Design review of the part shown in the three views and the two pictorial views. Dimensions are in mm from the part's minimum x, y and z. A direction names the side the tool comes from. Coordinates: 2 decimals unless noted, no trailing zeros. Loops run counter-clockwise (first coordinate to the right, second up) from the corner with the lowest first, then second, coordinate; pieces in that order, holes last. Notation, with made-up numbers: (28, 87.25) -> (53, 87.25) arc R21 cw to (53, 124.25) -> close; hole circle Ø6 at (47, 45.5). An arc over 180 degrees is marked (long way). One line per item, written item: value.
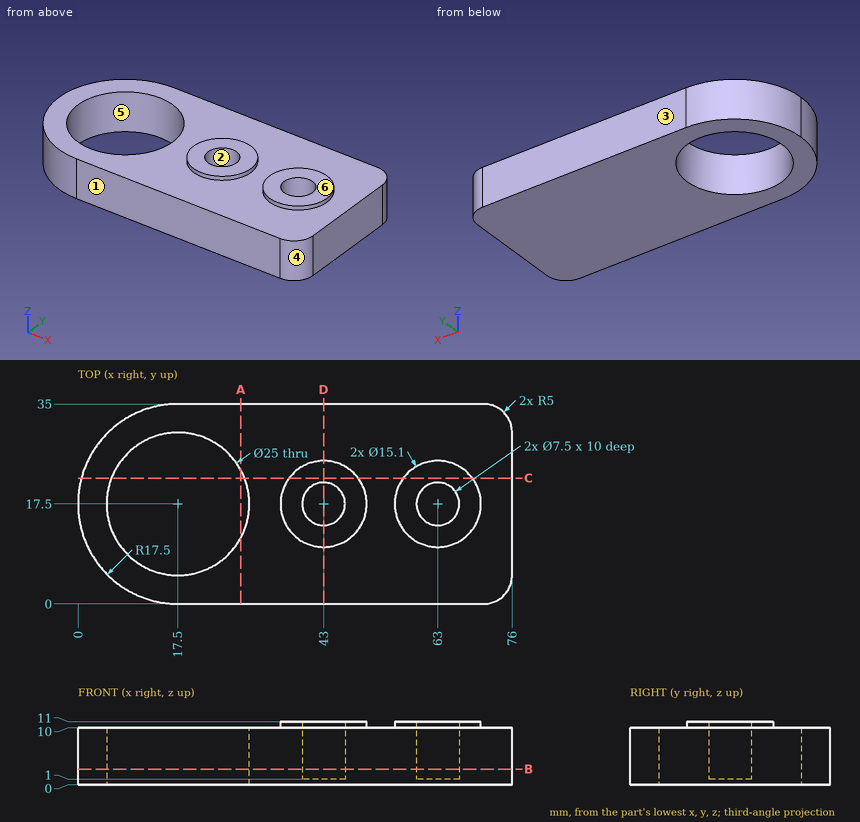
1. Insertion check: pin 1 Ø10.5 at (x, y) = (54, 11) entering from +Z; pin 2 Ø4 at (x, y) = (42.5, 18) entering from +Z; pin 3 Ø5 at (y, z) = (10.5, 3) entering from -X; pin 4 Ø6 at (y, z) = (11, 2) entering from -X. Each pin has a flat end and moves straight along its axis. Give the tip position at first contact, or say it passes through.
Return value:
pin 1: stops at z = 11
pin 2: stops at z = 1
pin 3: stops at x = 0.59
pin 4: stops at x = 0.35
2. Take a section at D-D, the plane x = 43. Give the boundary of the cut face in (y, z), and give its area (3 significant figures).
Return value:
outline: (0, 0) -> (35, 0) -> (35, 10) -> (25.05, 10) -> (25.05, 11) -> (21.25, 11) -> (21.25, 1) -> (13.75, 1) -> (13.75, 11) -> (9.95, 11) -> (9.95, 10) -> (0, 10) -> close
area: 290 mm2
3. The part is to be moulded in two halves that separate along Y. For the marked faces 3, 4, 5 and 6, say which applies: pulls with the +Y half, pulls with the -Y half, needs draft (parallel to the pull), parting line crosses it, or undercut.
Return value:
face 3: pulls with the +Y half
face 4: pulls with the -Y half
face 5: undercut
face 6: needs draft
4. Take a section at B-B, the plane z = 2.75. Give the boundary of the cut face in (x, y), and give its area (3 significant figures).
Return value:
outline: (17.5, 0) -> (71, 0) arc R5 ccw to (76, 5) -> (76, 30) arc R5 ccw to (71, 35) -> (17.5, 35) arc R17.5 ccw to start; hole circle Ø25 at (17.5, 17.5); hole circle Ø7.5 at (43, 17.5); hole circle Ø7.5 at (63, 17.5)
area: 1,940 mm2
5. To check wall thickness, follow probe 1 along Y at (x, z) = (43, 3.5); probe 2 along Y at (x, z) = (17.5, 3.75); probe 3 along X at (y, z) = (19, 3). State the ranges of each line that lie inside material, in increasing order. Write a range as from..to.
Return value:
probe 1: y = 0..13.75, 21.25..35
probe 2: y = 0..5, 30..35
probe 3: x = 0.06..5.09, 29.91..39.56, 46.44..59.56, 66.44..76
6. Take a section at C-C, the plane y = 22. Give the boundary of the cut face in (x, z), and give its area (3 significant figures).
Return value:
outline: (0.59, 0) -> (5.84, 0) -> (5.84, 10) -> (0.59, 10) -> close; (29.16, 0) -> (76, 0) -> (76, 10) -> (69.06, 10) -> (69.06, 11) -> (56.94, 11) -> (56.94, 10) -> (49.06, 10) -> (49.06, 11) -> (36.94, 11) -> (36.94, 10) -> (29.16, 10) -> close
area: 545 mm2
7. For the marked faces 1 and 2, list the 3-axis set-ups (+Z, -Z, +X, -X, +Y, -Y) from which the entire face can be reached by the end or side of a thin tool; tool diameter is ignored.
Return value:
face 1: +Z, -Z, +X, -X, -Y
face 2: +Z
8. Take a section at A-A, the plane x = 28.5. Give the boundary of the cut face in (y, z), and give its area (3 significant figures).
Return value:
outline: (0, 0) -> (11.56, 0) -> (11.56, 10) -> (0, 10) -> close; (23.44, 0) -> (35, 0) -> (35, 10) -> (23.44, 10) -> close
area: 231 mm2
